Autodesk Inventor part; units mm, degrees
ref_plane "YZ Plane" through (0, 0, 0) normal (1, 0, 0) x (0, 1, 0)
ref_plane "XZ Plane" through (0, 0, 0) normal (0, 1, 0) x (-1, 0, 0)
ref_plane "XY Plane" through (0, 0, 0) normal (0, 0, 1) x (1, 0, 0)
sketch "Sketch1" plane through (0, 0, 0) normal (0, 0, 1) x (1, 0, 0)
  line L0 (0, 0) -> (0, 10.0763) construction
  line L1 (11.1, 9) -> (11.1, 2)
  line L2 (11.1, 2) -> (9.1, 2)
  line L3 (9.1, 2) -> (9.1, 0)
  line L4 (9.1, 0) -> (14.875, 0)
  line L5 (14.875, 0) -> (14.875, 3)
  line L6 (14.875, 3) -> (13.26, 3)
  line L7 (13.26, 3) -> (13.26, 9)
  line L8 (13.26, 9) -> (11.1, 9)
  dimension "d0" = 2
  dimension "d1" = 7
  dimension "d2" = 13.26
  dimension "d3" = 14.875
  dimension "d4" = 6
  dimension "d5" = 11.1
  dimension "d6" = 2
revolve "Revolution1" add sketch "Sketch1" angle 360 about axis through (0, 0, 0) along (0, 1, 0)
fillet "Fillet1" radius 0.5 4 edges at (-13.26, 9, 0) (-11.1, 9, 0) (-14.875, 3, 0) (-9.1, 2, 0)
properties part number "beltPulley"
Verification items for the finished model (mm, model axes). A direction names the side the tool comes from. Coordinates: 2 decimals unless noted, no trailing zeros. Loops run counter-clockwise (first coordinate to the right, second up) from the corner with the lowest first, then second, coordinate; pieces in that order, holes last. Notation, with made-up numbers: (-18.75, -12) - (27.25, -12) arc R7 cw to (27.25, -7) - close; hole circle Ø11 at (18, 74). An arc over 180 degrees is marked (long way). Put each result on its own line as item: value.
Item 1: Scan lines: line 1 along X through (y, z) = (0.7, 0) (3 decimals); line 2 along Z through (x, y) = (0, 7.25). Record each from-to range of solid material in increasing order.
Conclusion:
line 1: x = -14.875 to -9.1, 9.1 to 14.875
line 2: z = -13.26 to -11.1, 11.1 to 13.26
Item 2: Set-up check for faces 4 (the face through (5.61, 9, 10.34)), 5 (the face through (-7, 2, -7)): record each of +Z, -Z, +X, -X, +Y, -Y from which the full face is reachable in a straight line by a thin tool's end or side.
Conclusion:
face 4: +Z, -Z, +X, -X, +Y
face 5: +Y
Item 3: Gauge pin test, flat ends, axial feed: pin 1 Ø6.5 at (x, z) = (2.5, -1) entering from +Y; pin 2 Ø1.5 at (x, y) = (10, 3) entering from +Z; pin 3 Ø5 at (x, y) = (-4, 4.5) entering from -Z; pin 4 Ø3 at (x, y) = (-8.5, 3.5) entering from +Z. Record the tip position at first contact, or that the pin passes through.
Conclusion:
pin 1: passes through
pin 2: stops at z = 11.55
pin 3: stops at z = -14.67
pin 4: stops at z = 12.95
Item 4: Section check C-C (y = 1). Enter the section's corners in (x, z) (3 decimals), then the cut area to 3 significant figures.
Conclusion:
outline: circle Ø29.75 at (0, 0); hole circle Ø18.2 at (0, 0)
area: 435 mm2
Item 5: Section check A-A (x = 0). Enter the section's corners in (y, z) (3 decimals), then the cut area to 3 significant figures.
Conclusion:
outline: (0, -14.875) - (2.5, -14.875) arc R0.5 ccw to (3, -14.375) - (3, -13.26) - (8.5, -13.26) arc R0.5 ccw to (9, -12.76) - (9, -11.6) arc R0.5 ccw to (8.5, -11.1) - (2, -11.1) - (2, -9.6) arc R0.5 ccw to (1.5, -9.1) - (0, -9.1) - close; (0, 9.1) - (1.5, 9.1) arc R0.5 ccw to (2, 9.6) - (2, 11.1) - (8.5, 11.1) arc R0.5 ccw to (9, 11.6) - (9, 12.76) arc R0.5 ccw to (8.5, 13.26) - (3, 13.26) - (3, 14.375) arc R0.5 ccw to (2.5, 14.875) - (0, 14.875) - close
area: 56.1 mm2
Item 6: Draft check along X on faces 1 (the face through (-2.875, 5.788, 12.945)), 2 (the face through (4, 3, 13)), 3 (the face through (5.97, 5.2, 9.36)). Enter one of: pulls with the +X half, pulls with the -X half, needs draft (parallel to the pull), parting line crosses it, or undercut.
Conclusion:
face 1: parting line crosses it
face 2: needs draft
face 3: undercut
Item 7: Section check B-B (z = 0). Enter the section's corners in (x, y) (3 decimals), then the cut area to 3 significant figures.
Conclusion:
outline: (-14.875, 0) - (-9.1, 0) - (-9.1, 1.5) arc R0.5 ccw to (-9.6, 2) - (-11.1, 2) - (-11.1, 8.5) arc R0.5 ccw to (-11.6, 9) - (-12.76, 9) arc R0.5 ccw to (-13.26, 8.5) - (-13.26, 3) - (-14.375, 3) arc R0.5 ccw to (-14.875, 2.5) - close; (9.1, 0) - (14.875, 0) - (14.875, 2.5) arc R0.5 ccw to (14.375, 3) - (13.26, 3) - (13.26, 8.5) arc R0.5 ccw to (12.76, 9) - (11.6, 9) arc R0.5 ccw to (11.1, 8.5) - (11.1, 2) - (9.6, 2) arc R0.5 ccw to (9.1, 1.5) - close
area: 56.1 mm2
